from build123d import *

# Parameters (mm, degrees)
SKETCH1_R               = 22.5
BOSS_EXTRUDE1_DEPTH     = 3
SKETCH2_R               = 5
BOSS_EXTRUDE2_DEPTH     = 70
SKETCH3_R               = 12
BOSS_EXTRUDE3_DEPTH     = 28
FILLET1_R               = 6
CUT_EXTRUDE1_DEPTH      = 80.633535649
CUT_EXTRUDE1_DEPTH_BACK = 80.633535649
SKETCH4_W               = 19.57
SKETCH4_H               = 20


with BuildPart() as part:
    # Sketch1 → Boss-Extrude1 (new body)
    with BuildSketch(Plane(origin=(0, 0, 0), x_dir=(1, 0, 0), z_dir=(0, 1, 0))):
        with Locations(Location((0, 0, 0), (0, 0, 270))):
            Circle(SKETCH1_R)
    extrude(amount=BOSS_EXTRUDE1_DEPTH)

    # Sketch2 → Boss-Extrude2 (add)
    with BuildSketch(Plane(origin=(0, 3, 0), x_dir=(1, 0, 0), z_dir=(0, 1, 0))):
        with Locations(Location((0, 0, 0), (0, 0, 270))):
            Circle(SKETCH2_R)
    extrude(amount=BOSS_EXTRUDE2_DEPTH)

    # Sketch3 → Boss-Extrude3 (add)
    with BuildSketch(Plane.XZ):
        with Locations(Location((0, 0, 0), (0, 0, 270))):
            Circle(SKETCH3_R)
    extrude(amount=BOSS_EXTRUDE3_DEPTH)

    # Fillet1
    fillet1_edges = [part.edges().sort_by_distance(p)[0] for p in [
        (0, -28, 12),
    ]]
    fillet(fillet1_edges, radius=FILLET1_R)

    # Sketch4 → Cut-Extrude1 (cut, two sides: drawn at the far end of the back side and taken through both)
    with BuildSketch(Plane.XY.offset(-CUT_EXTRUDE1_DEPTH_BACK)):
        with Locations((17.285, -18)):
            Rectangle(SKETCH4_W, SKETCH4_H)
        with Locations((-17.285, -18)):
            Rectangle(SKETCH4_W, SKETCH4_H)
    extrude(amount=CUT_EXTRUDE1_DEPTH + CUT_EXTRUDE1_DEPTH_BACK, mode=Mode.SUBTRACT)


solid = part.part
Verification items for the finished model (mm, model axes). A direction names the side the tool comes from. Coordinates: 2 decimals unless noted, no trailing zeros. Order: outer loops, then holes, each group sorted by start corner. A loop starts at its lowest first (then second) coordinate and runs counter-clockwise, first axis right, second up. Notation, with made-up numbers: M 69,61 L 74,61 A18 ccw 74,83 Z; hole C 77.25,-23.5 d4. An arc over 180 degrees is marked long. One line per item, written item: value. Start each with the question number.
Item 1: Sectioned sample at B-B (y = -4.5). Enter the section's corners in (x, z).
Item 2: Access from +Z, -Z, +X, -X, +Y, -Y to the whole of each face (thin tool, end or side, straight path). Record for faces 1 (the flat face through (9, -8, 0)), 2 (the cylindrical face through (-8.618, 1.479, 20.784)), 3 (the flat face through (-7.5, -18, 0)), 4 (the cylindrical face through (-4.88, 37.51, -1.08)), 5 (the cylindrical face through (-11.715, -5.957, 2.601)).
Item 3: Gauge pin test, flat ends, axial feed: pin 1 (3.5 mm diameter, centred on x = 10.5, z = 1, fed in from -Y); pin 2 (1.5 mm diameter, centred on x = 6.5, y = 62, fed in from +Z); pin 3 (8 mm diameter, centred on x = 6, z = 10.5, fed in from -Y); pin 4 (12 mm diameter, centred on y = 59.5, z = -3, fed in from -X). Record the tip position at first contact, or that the pin passes through.
Item 4: Scan lines: probe 1 along Y at (x, z) = (9, -17); probe 2 along Y at (x, z) = (1, 5); probe 3 along X at (y, z) = (52, 0). Record each from-to range of solid material in increasing order.
Item 5: Sectioned sample at A-A (x = 10). Enter the section's corners in (y, z), then the cut area to 3 significant figures.
Item 6: Sectioned sample at D-D (z = -17). Enter the section's corners in (x, y).
Item 7: Sectioned sample at C-C (z = 16.5). Enter the section's corners in (x, y), then the cut area to 3 significant figures.
Conclusion:
1. outline: C 0,0 d24
2. face 1: +Z, -Z, +X, -Y
2. face 2: +Y, -Y
2. face 3: +Z, -Z, -X, -Y
2. face 4: +Y
2. face 5: -Y
3. pin 1: stops at y = -8
3. pin 2: passes through
3. pin 3: stops at y = -27.62
3. pin 4: stops at x = -5
4. probe 1: y = 0 to 3
4. probe 2: y = -28 to 3
4. probe 3: x = -5 to 5
5. outline: M -8,-6.63 L 0,-6.63 L 0,-20.16 L 3,-20.16 L 3,20.16 L 0,20.16 L 0,6.63 L -8,6.63 Z
5. area: 227 mm^2
6. outline: M -14.74,0 L 14.74,0 L 14.74,3 L -14.74,3 Z
7. outline: M -15.3,0 L 15.3,0 L 15.3,3 L -15.3,3 Z
7. area: 91.8 mm^2
